from build123d import *

# Parameters (mm, degrees)
SKETCH1_R           = 7.5
SKETCH1_R_2         = 5
BOSS_EXTRUDE1_DEPTH = 4
SKETCH2_R           = 7
SKETCH2_R_2         = 5.5
CUT_EXTRUDE1_DEPTH  = 0.5


with BuildPart() as part:
    # Sketch1 → Boss-Extrude1 (new body)
    with BuildSketch(Plane(origin=(0, 0, 0), x_dir=(1, 0, 0), z_dir=(0, 1, 0))):
        Circle(SKETCH1_R)
        Circle(SKETCH1_R_2, mode=Mode.SUBTRACT)
    extrude(amount=BOSS_EXTRUDE1_DEPTH)

    # Sketch2 → Cut-Extrude1 (cut)
    with BuildSketch(Plane(origin=(0, 4, 0), x_dir=(1, 0, 0), z_dir=(0, 1, 0))):
        Circle(SKETCH2_R)
        Circle(SKETCH2_R_2, mode=Mode.SUBTRACT)
    cut_extrude1 = extrude(amount=-CUT_EXTRUDE1_DEPTH, mode=Mode.SUBTRACT)

    # Mirror1: Cut-Extrude1 across plane
    add(cut_extrude1.mirror(Plane(origin=(0, 2, 0), x_dir=(0, 0, 1), z_dir=(0, -1, 0))), mode=Mode.SUBTRACT)


solid = part.part
Source: CAD feature listing. Evaluate the final solid. Frame: model axes, mm. A direction names the side the tool comes from. Coordinates: 2 decimals unless noted, no trailing zeros. Loops run counter-clockwise (first coordinate to the right, second up) from the corner with the lowest first, then second, coordinate; pieces in that order, holes last. Notation, with made-up numbers: M 12.5,-34 L 65.5,-34 A22 cw 65.5,4 Z; hole C -10,10 d3. An arc over 180 degrees is marked long. Answer in a Markdown table with one row per item.
Q1. Section C-C on y = 0.9. Return the cut outline in (x, z).
Answers below:
| item | result |
|---|---|
| outline | C 0,0 d15; hole C 0,0 d10 |
Q2. Section A-A on x = 0. Return the cut outline in (y, z), plus the area to 3 significant figures.
Answers below:
| item | result |
|---|---|
| outline | M 0,-7.5 L 4,-7.5 L 4,-7 L 3.5,-7 L 3.5,-5.5 L 4,-5.5 L 4,-5 L 0,-5 L 0,-5.5 L 0.5,-5.5 L 0.5,-7 L 0,-7 Z; M 0,5 L 4,5 L 4,5.5 L 3.5,5.5 L 3.5,7 L 4,7 L 4,7.5 L 0,7.5 L 0,7 L 0.5,7 L 0.5,5.5 L 0,5.5 Z |
| area | 17.0 mm^2 |
Q3. Ray query, probe 1 along Z at (x, y) = (0, 0.45); probe 2 along X at (y, z) = (3, 0). Return the intervals inside material, ascending. Write a range as from..to.
Answers below:
| item | result |
|---|---|
| probe 1 | z = -7.5..-7, -5.5..-5, 5..5.5, 7..7.5 |
| probe 2 | x = -7.5..-5, 5..7.5 |
Q4. Draft query along X for faces 4 (the flat face through (7, 0, -2)), 5 (the cylindrical face through (-7.493, 1.972, -0.33)), 6 (the cylindrical face through (-1.19, 0.25, 5.37)). Return one class per face: pulls with the +X half, pulls with the -X half, needs draft (parallel to the pull), parting line crosses it, or undercut.
Answers below:
| item | result |
|---|---|
| face 4 | needs draft |
| face 5 | parting line crosses it |
| face 6 | undercut |
Q5. Section B-B on z = 0. Return the cut outline in (x, y).
Answers below:
| item | result |
|---|---|
| outline | M -7.5,0 L -7,0 L -7,0.5 L -5.5,0.5 L -5.5,0 L -5,0 L -5,4 L -5.5,4 L -5.5,3.5 L -7,3.5 L -7,4 L -7.5,4 Z; M 5,0 L 5.5,0 L 5.5,0.5 L 7,0.5 L 7,0 L 7.5,0 L 7.5,4 L 7,4 L 7,3.5 L 5.5,3.5 L 5.5,4 L 5,4 Z |
Q6. First-contact query: pin 1 (2 mm diameter, centred on y = 1.5, z = -5.5, fed in from -X); pin 2 (1 mm diameter, centred on y = 3.5, z = -6, fed in from -X). Flat tips, straight axial feed; report the tip coordinate or a pass-through.
Answers below:
| item | result |
|---|---|
| pin 1 | stops at x = -6 |
| pin 2 | stops at x = -5.1 |
Q7. Section D-D on z = 6.25. Return the cut outline in (x, y), plus the area to 3 significant figures.
Answers below:
| item | result |
|---|---|
| outline | M -4.15,0 L -3.15,0 L -3.15,0.5 L 3.15,0.5 L 3.15,0 L 4.15,0 L 4.15,4 L 3.15,4 L 3.15,3.5 L -3.15,3.5 L -3.15,4 L -4.15,4 Z |
| area | 26.9 mm^2 |
Q8. Set-up query: faces 1 (the flat face through (7, 4, -2)), 2 (the cylindrical face through (6.466, 0.246, 2.681)), 3 (the cylindrical face through (-1.19, 3.75, 5.37)). Return all of +Z, -Z, +X, -X, +Y, -Y with unobstructed straight access to the full face (end or side cutting, diameter ignored); none if empty.
Answers below:
| item | result |
|---|---|
| face 1 | +Z, -Z, +X, -X, +Y |
| face 2 | -Y |
| face 3 | +Y |
